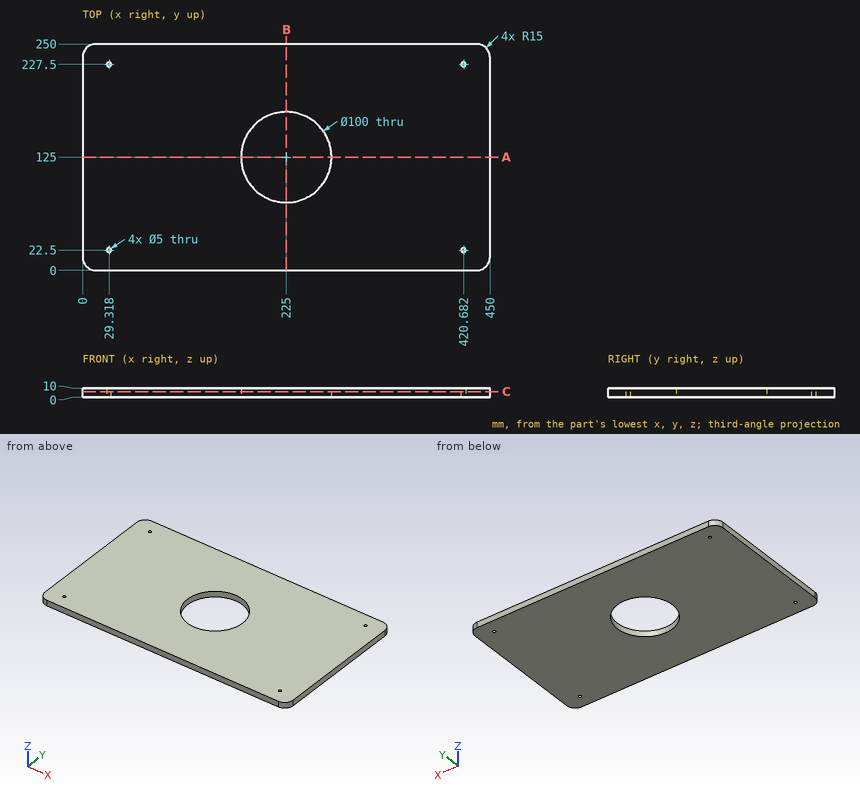
Print and shaded views of the part. All mm, measured from the part's lowest x, y and z. Give positions to 0.01 mm unless a question says otherwise; leave off trailing zeros. Loops run counter-clockwise (first coordinate to the right, second up) from the corner with the lowest first, then second, coordinate; pieces in that order, holes last. Notation, with made-up numbers: (29.25, 16.25) -> (57.25, 16.25) arc R21 ccw to (57.25, 36.25) -> close; hole circle Ø2 at (65, 55.25). An arc over 180 degrees is marked (long way). Use CSV: the item, a comma, the result in double quotes. Start each with the question number.
1) Slice it at A-A on y = 125. Give the cut face in (x, z).
2) Flat gauge pins, fed straight in: pin 1 Ø4.5 at (x, y) = (420.68, 22.5) entering from -Z; pin 2 Ø12 at (x, y) = (391, 66) entering from -Z. Where does each tip first touch, or does it go through?
3) Slice it at C-C on z = 6.5. Give the cut face in (x, y).
4) Wall check: line 1 (X direction, y = 227.5, z = 2.5); line 2 (X direction, y = 124.5, z = 5.5); line 3 (Y direction, x = 194, z = 7). Give the ranges that are in metal, low to high.
5) Slice it at B-B on x = 225. Give the cut face in (y, z).
Computed values:
1,outline,"(0, 0) -> (175, 0) -> (175, 10) -> (0, 10) -> close; (275, 0) -> (450, 0) -> (450, 10) -> (275, 10) -> close"
2,pin 1,"passes through"
2,pin 2,"stops at z = 0"
3,outline,"(0, 15) arc R15 ccw to (15, 0) -> (435, 0) arc R15 ccw to (450, 15) -> (450, 235) arc R15 ccw to (435, 250) -> (15, 250) arc R15 ccw to (0, 235) -> close; hole circle Ø5 at (29.32, 22.5); hole circle Ø5 at (29.32, 227.5); hole circle Ø100 at (225, 125); hole circle Ø5 at (420.68, 22.5); hole circle Ø5 at (420.68, 227.5)"
4,line 1,"x = 0 to 26.82, 31.82 to 418.18, 423.18 to 450"
4,line 2,"x = 0 to 175, 275 to 450"
4,line 3,"y = 0 to 85.77, 164.23 to 250"
5,outline,"(0, 0) -> (75, 0) -> (75, 10) -> (0, 10) -> close; (175, 0) -> (250, 0) -> (250, 10) -> (175, 10) -> close"
